```python
from build123d import *

# Parameters (mm, degrees)
BOSS_EXTRUDE1_DEPTH = 60
SKETCH2_R           = 2
BOSS_EXTRUDE2_DEPTH = 30


with BuildPart() as part:
    # Sketch1 → Boss-Extrude1 (new body)
    with BuildSketch(Plane(origin=(0, 0, 0), x_dir=(1, 0, 0), z_dir=(0, 1, 0))):
        Polygon((-15, 5), (-14.049599683, 5), (-14.049599683, 3), (-11.049599683, 3), (-11.049599683, 5), (-9.049599683, 5), (-9.049599683, 3), (-6.049599683, 3), (-6.049599683, 5), (-4.049599683, 5), (-4.049599683, 3), (-1.049599683, 3), (-1.049599683, 5), (0.950400317, 5), (0.950400317, 3), (3.950400317, 3), (3.950400317, 5), (5.950400317, 5), (5.950400317, 3), (8.950400317, 3), (8.950400317, 5), (10.950400317, 5), (10.950400317, 3), (13.950400317, 3), (13.950400317, 5), (15, 5), (15, -5), (-15, -5), align=None)
    extrude(amount=BOSS_EXTRUDE1_DEPTH)

    # Sketch2 → Boss-Extrude2 (add)
    with BuildSketch(Plane.XZ):
        with Locations(Location((0, 0, 0), (0, 0, 90))):
            Circle(SKETCH2_R)
        with Locations(Location((10, 0, 0), (0, 0, 90))):
            Circle(SKETCH2_R)
        with Locations(Location((-10, 0, 0), (0, 0, 90))):
            Circle(SKETCH2_R)
    extrude(amount=BOSS_EXTRUDE2_DEPTH)


solid = part.part
```
Can you work these out from the model? Positions are in its coordinate system, mm. A direction names the side the tool comes from. Coordinates: 2 decimals unless noted, no trailing zeros. Order: outer loops, then holes, each group sorted by start corner. A loop starts at its lowest first (then second) coordinate and runs counter-clockwise, first axis right, second up. Notation, with made-up numbers: (58, 73) - (77, 73) arc R8 cw to (77, 77) - close; hole circle Ø4 at (-24.75, 17.5). An arc over 180 degrees is marked (long way). Answer in a Markdown table with one row per item.
1. If I drill on line 1 along X through (y, z) = (-19, 0); line 2 along Y through (x, z) = (-8.5, -2.75); line 3 along Z through (x, y) = (2.5, 48), over which ranges is the centre line in solid material (lowest first)?
Reply:
| item | result |
|---|---|
| line 1 | x = -12 to -8, -2 to 2, 8 to 12 |
| line 2 | y = 0 to 60 |
| line 3 | z = -3 to 5 |
2. Suppose I cut it at D-D (z = 0). Please give me the cut outline in (x, y).
Reply:
| item | result |
|---|---|
| outline | (-15, 0) - (-12, 0) - (-12, -30) - (-8, -30) - (-8, 0) - (-2, 0) - (-2, -30) - (2, -30) - (2, 0) - (8, 0) - (8, -30) - (12, -30) - (12, 0) - (15, 0) - (15, 60) - (-15, 60) - close |
3. For faces 4 (the flat face through (0, 60, 1)), 5 (the flat face through (-13, 30, -3)), 6 (the cylindrical face through (2, -15, 0)), which set-ups out of +Z, -Z, +X, -X, +Y, -Y let a thin tool reach every point of the face, with its end or its side?
Reply:
| item | result |
|---|---|
| face 4 | +Z, -Z, +X, -X, +Y |
| face 5 | -Z, +Y, -Y |
| face 6 | -Y |
4. Suppose I cut it at C-C (y = -14). Please give me the cut outline in (x, z).
Reply:
| item | result |
|---|---|
| outline | circle Ø4 at (-10, 0); circle Ø4 at (0, 0); circle Ø4 at (10, 0) |
5. Suppose I cut it at B-B (x = -10). Please give me the cut outline in (y, z).
Reply:
| item | result |
|---|---|
| outline | (-30, -2) - (0, -2) - (0, -5) - (60, -5) - (60, 5) - (0, 5) - (0, 2) - (-30, 2) - close |
6. If we mould it in two halves opening along X, with no side actions, what happens to faces 1 (the flat face through (3.95, 30, -4)), 2 (the flat face through (-10, 30, -5)), 3 (the flat face through (15, 30, 0))? For each: pulls with the +X half, pulls with the -X half, needs draft (parallel to the pull), parting line crosses it, or undercut.
Reply:
| item | result |
|---|---|
| face 1 | undercut |
| face 2 | needs draft |
| face 3 | pulls with the +X half |
7. For pin 1 (1.5 mm diameter, centred on x = 7.5, y = 30.5, fed in from -Z); pin 2 (4 mm diameter, centred on y = -15, z = -1.5, fed in from -X), each with a flat end and sliding along its axis, tell me the tip position at first contact or that it passes through.
Reply:
| item | result |
|---|---|
| pin 1 | stops at z = -3 |
| pin 2 | stops at x = -12 |
8. Suppose I cut it at A-A (z = -4). Please give me the cut outline in (x, y).
Reply:
| item | result |
|---|---|
| outline | (-15, 0) - (-14.05, 0) - (-14.05, 60) - (-15, 60) - close; (-11.05, 0) - (-9.05, 0) - (-9.05, 60) - (-11.05, 60) - close; (-6.05, 0) - (-4.05, 0) - (-4.05, 60) - (-6.05, 60) - close; (-1.05, 0) - (0.95, 0) - (0.95, 60) - (-1.05, 60) - close; (3.95, 0) - (5.95, 0) - (5.95, 60) - (3.95, 60) - close; (8.95, 0) - (10.95, 0) - (10.95, 60) - (8.95, 60) - close; (13.95, 0) - (15, 0) - (15, 60) - (13.95, 60) - close |
